Can you work these out from the model? Positions are in its coordinate system, mm. Face numbers are marked on the shaded views. A direction names the side the tool comes from. Give positions to 0.01 mm unless a question says otherwise; leave off trailing zeros. Loops run counter-clockwise (first coordinate to the right, second up) from the corner with the lowest first, then second, coordinate; pieces in that order, holes last. Notation, with made-up numbers: (-30, -13.5) - (11, -13.5) arc R34 ccw to (11, 17.5) - close; hole circle Ø3 at (35.25, 14.5). An arc over 180 degrees is marked (long way). Answer in a Markdown table with one row per item.
Autodesk Inventor part; units mm, degrees
ref_plane "YZ Plane" through (0, 0, 0) normal (1, 0, 0) x (0, 1, 0)
ref_plane "XZ Plane" through (0, 0, 0) normal (0, 1, 0) x (-1, 0, 0)
ref_plane "XY Plane" through (0, 0, 0) normal (0, 0, 1) x (1, 0, 0)
sketch "Sketch1" plane through (0, 0, 0) normal (0, 1, 0) x (-1, 0, 0)
  line L0 (0, 0) -> (50, 0)
  line L1 (50, 0) -> (50, -30)
  line L2 (50, -30) -> (0, -30)
  line L3 (0, -30) -> (0, 0)
  dimension "d0" = 50
  dimension "d1" = 30
extrude "Extrusion1" add sketch "Sketch1" along normal blind 50
sketch "Sketch2" plane through (0, 50, 0) normal (0, 1, 0) x (1, 0, 0)
  line L0 (5, -5) -> (-55, -5)
  line L1 (-55, -5) -> (-55, 35)
  line L2 (-55, 35) -> (5, 35)
  line L3 (5, 35) -> (5, -5)
  point P0 (0, 0)
  dimension "d4" = 60
  dimension "d5" = 40
extrude "Extrusion2" add sketch "Sketch2" against normal blind 30
sketch "Sketch3" plane through (0, 50, 0) normal (0, 1, 0) x (1, 0, 0)
  line L0 (0, 0) -> (0, 30)
  line L1 (0, 30) -> (-50, 30)
  line L2 (0, 0) -> (-50, 0)
  line L3 (-50, 0) -> (-50, 30)
  line L4 (-50, 30) -> (0, 30)
  line L5 (0, 30) -> (0, 0)
  line L6 (5, -5) -> (-55, -5)
  line L7 (-55, -5) -> (-55, 35)
  line L8 (5, -5) -> (-55, -5)
  line L9 (-55, -5) -> (-55, 35)
  line L10 (-55, 35) -> (5, 35)
  line L11 (5, 35) -> (5, -5)
  dimension "d8" = 50
  dimension "d9" = 30
extrude "Extrusion3" cut sketch "Sketch3" against normal blind 28
sketch "Sketch4" plane through (0, 0, 0) normal (0, -1, 0) x (1, 0, 0)
  line L0 (-50, 0) -> (0, 0)
  line L1 (0, -30) -> (-50, -30)
  line L2 (0, 0) -> (-50, 0)
  line L3 (-50, 0) -> (-50, -30)
  line L4 (-50, -30) -> (0, -30)
  line L5 (0, -30) -> (0, 0)
extrude "Extrusion4" cut sketch "Sketch4" against normal blind 5
sketch "Sketch5" plane through (0, 5, 0) normal (0, -1, 0) x (1, 0, 0)
  circle A0 centre (-25, -15) radius 2.5
  point P0 (0, 0)
  dimension "d14" = 5
extrude "Extrusion5" add sketch "Sketch5" along normal blind 3
sketch "Sketch6" plane through (-25, 2, -15) normal (0, -1, 0) x (1, 0, 0)
  line L0 (-12.5, 12.5) -> (12.5, 12.5)
  line L1 (12.5, 12.5) -> (12.5, -12.5)
  line L2 (12.5, -12.5) -> (-12.5, -12.5)
  line L3 (-12.5, -12.5) -> (-12.5, 12.5)
  circle A0 centre (-10, 10) radius 1.5
  circle A1 centre (-10, -10) radius 1.5
  circle A2 centre (10, -10) radius 1.5
  circle A3 centre (10, 10) radius 1.5
  point P0 (25, 15)
  dimension "d19" = 25
  dimension "d20" = 25
  dimension "d21" = 3
  dimension "d22" = 3
  dimension "d23" = 3
  dimension "d24" = 3
extrude "Extrusion6" add sketch "Sketch6" along normal blind 2
sketch "Sketch7" plane through (-25, 0, -15) normal (0, -1, 0) x (1, 0, 0)
  circle A0 centre (0, 0) radius 2.5
  point P0 (25, 15)
  dimension "d27" = 5
extrude "Extrusion7" add sketch "Sketch7" along normal blind 3
sketch "Sketch8" plane through (0, 20, 0) normal (0, -1, 0) x (1, 0, 0)
  line L0 (-50, -30) -> (-50, 0)
  circle A0 centre (-5, -32.5) radius 1.5
  circle A1 centre (-5, 2.5) radius 1.5
  circle A2 centre (-45, 2.5) radius 1.5
  circle A3 centre (-45, -32.5) radius 1.5
  point P0 (0, 0)
  point P1 (0, -30)
  dimension "d38" = 3
  dimension "d39" = 3
  dimension "d40" = 3
  dimension "d41" = 3
extrude "Extrusion8" cut sketch "Sketch8" against normal blind 3
properties part number "Servo"
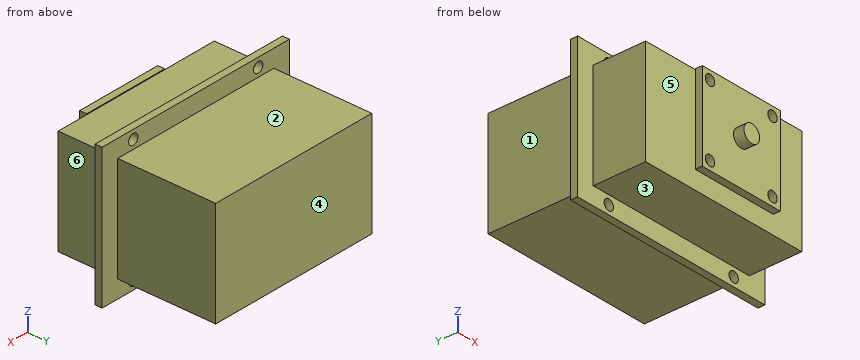
Q1. For pin 1 (6 mm diameter, centred on y = 13.5, z = -13.5, fed in from +X); pin 2 (0.6 mm diameter, centred on x = -19, y = 1, fed in from +Z); pin 3 (4.5 mm diameter, centred on x = -29.5, y = 13.5, fed in from -Z); pin 4 (7.5 mm diameter, centred on x = -22, z = -12.5, fed in from -Y), each with a flat end and sliding along its axis, tell me the tip position at first contact or that it passes through.
Checked values:
| item | result |
|---|---|
| pin 1 | stops at x = 0 |
| pin 2 | stops at z = -2.5 |
| pin 3 | stops at z = -30 |
| pin 4 | stops at y = -3 |
Q2. Imagine slicing it at B-B, the plane z = -5. Write out the boundary of the cut face in (x, y), and give its area (3 significant figures).
Checked values:
| item | result |
|---|---|
| outline | (-55, 20) - (-50, 20) - (-50, 5) - (0, 5) - (0, 20) - (5, 20) - (5, 22) - (0, 22) - (0, 50) - (-50, 50) - (-50, 22) - (-55, 22) - close; (-37.5, 0) - (-36.5, 0) - (-36.5, 2) - (-37.5, 2) - close; (-33.5, 0) - (-16.5, 0) - (-16.5, 2) - (-33.5, 2) - close; (-13.5, 0) - (-12.5, 0) - (-12.5, 2) - (-13.5, 2) - close |
| area | 2,310 mm² |
Q3. If we mould it in two halves opening along Y, with no side actions, what happens to the marked faces 4, 5 and 6? For each: released by +Y, released by -Y, zero draft, split by the parting line, or undercut.
Checked values:
| item | result |
|---|---|
| face 4 | released by +Y |
| face 5 | undercut |
| face 6 | zero draft |
Q4. Imagine slicing it at C-C, the plane x = -35. Write out the boundary of the cut face in (y, z), and give its area (3 significant figures).
Checked values:
| item | result |
|---|---|
| outline | (0, -27.5) - (2, -27.5) - (2, -26.5) - (0, -26.5) - close; (0, -23.5) - (2, -23.5) - (2, -6.5) - (0, -6.5) - close; (0, -3.5) - (2, -3.5) - (2, -2.5) - (0, -2.5) - close; (5, -30) - (20, -30) - (20, -35) - (22, -35) - (22, -30) - (50, -30) - (50, 0) - (22, 0) - (22, 5) - (20, 5) - (20, 0) - (5, 0) - close |
| area | 1,410 mm² |
Q5. If I drill on line 1 (Z direction, x = -45, y = 21); line 2 (Y direction, x = -20.5, z = -13.5); line 3 (X direction, y = 9.5, z = -25), over which ranges is the centre line in solid material (lowest first)? Write a range as [from, to].
Checked values:
| item | result |
|---|---|
| line 1 | z = [-35, -34], [-31, 1], [4, 5] |
| line 2 | y = [0, 2], [5, 50] |
| line 3 | x = [-50, 0] |
Q6. Imagine slicing it at D-D, the plane z = -32.5. Write out the boundary of the cut face in (x, y).
Checked values:
| item | result |
|---|---|
| outline | (-55, 20) - (-46.5, 20) - (-46.5, 22) - (-55, 22) - close; (-43.5, 20) - (-6.5, 20) - (-6.5, 22) - (-43.5, 22) - close; (-3.5, 20) - (5, 20) - (5, 22) - (-3.5, 22) - close |
Q7. Imagine slicing it at A-A, the plane x = -45. Write out the boundary of the cut face in (y, z).
Checked values:
| item | result |
|---|---|
| outline | (5, -30) - (20, -30) - (20, -31) - (22, -31) - (22, -30) - (50, -30) - (50, 0) - (22, 0) - (22, 1) - (20, 1) - (20, 0) - (5, 0) - close; (20, -35) - (22, -35) - (22, -34) - (20, -34) - close; (20, 4) - (22, 4) - (22, 5) - (20, 5) - close |
Q8. On a 3-axis mill with a long thin cutter (end or side, diameter ignored), from which of +Z, -Z, +X, -X, +Y, -Y can I reach the whole of each face in a straight line? I mean the marked faces 1, 2 and 3. Say none if no direction works.
Checked values:
| item | result |
|---|---|
| face 1 | +Z, -Z, -X, +Y |
| face 2 | +Z, +X, -X, +Y |
| face 3 | -Z, +X, -X, -Y |
